Design review of the part built by this model. Coordinates are the model's own, in mm. A direction names the side the tool comes from. Give positions to 0.01 mm unless a question says otherwise; leave off trailing zeros. Write each loop counter-clockwise with the first axis right and the second up, starting at its lowest first coordinate (ties: lowest second). Pieces come first, ordered by that corner, then holes. Notation, with made-up numbers: (60, 77) -> (65, 77) arc R19 ccw to (65, 92) -> close; hole circle Ø6 at (-29.75, 11). An arc over 180 degrees is marked (long way). Return JSON: item names as keys, results as strings. Group by question number.
from build123d import *

# Parameters (mm, degrees)
F0_R     = 1.5
F0_R_2   = 13.666943
F1_DEPTH = 3
F0_W     = 3.25
F0_H     = 5.5
F0_W_2   = 17.75
F2_DEPTH = 45


with BuildPart() as f1:
    # F0 (on Top) → F1 (new body)
    with BuildSketch(Plane.XY):
        Polygon((21, 21), (-21, 21), (-21, -21), (-3.25, -21), (0, -21), (3.25, -21), (21, -21), align=None)
        with Locations((-15.5, -15.5)):
            Circle(F0_R, mode=Mode.SUBTRACT)
        with Locations((15.5, -15.5)):
            Circle(F0_R, mode=Mode.SUBTRACT)
        with Locations((-15.5, 15.5)):
            Circle(F0_R, mode=Mode.SUBTRACT)
        Circle(F0_R_2, mode=Mode.SUBTRACT)
        with Locations((15.5, 15.5)):
            Circle(F0_R, mode=Mode.SUBTRACT)
    extrude(amount=F1_DEPTH)

    # F0 (on Top) → F2 (join)
    with BuildSketch(Plane.XY):
        Polygon((0, -26.5), (-3.25, -26.5), (-3.25, -29.5), (-8.25, -29.5), (-5.5, -34), (0, -34), align=None)
        Polygon((3.25, -29.5), (3.25, -26.5), (0, -26.5), (0, -34), (5.5, -34), (8.25, -29.5), align=None)
        with Locations((1.625, -23.75)):
            Rectangle(F0_W, F0_H)
        with Locations((12.125, -23.75)):
            Rectangle(F0_W_2, F0_H)
        with Locations((-1.625, -23.75)):
            Rectangle(F0_W, F0_H)
        with Locations((-12.125, -23.75)):
            Rectangle(F0_W_2, F0_H)
    extrude(amount=F2_DEPTH)


solid = f1.part
Q1. Tool access review of faces 1 (the face through (-17, -15.43, 1.48)), 2 (the face through (12, -26.5, 22)), 3 (the face through (-12, -26.5, 22)), 4 (the face through (0, 14, 3)): name each direction out of +Z, -Z, +X, -X, +Y, -Y from which nothing blocks a thin tool from reaching the whole face with its end or side.
Q2. Take a section at C-C, the plane x = 0. Give the boundary of the cut face in (y, z), plus the area to 3 significant figures.
Q3. Mouldability with a two-part tool opening along Y and no side actions: class faces 5 (the face through (6.856, -31.782, 22.185)), 6 (the face through (0, -21, 24)), 7 (the face through (-10, -12, 0)), 8 (the face through (3.25, -28, 22)) as +Y half, -Y half, draft (parallel to the pull), parting line (faces both ways), or undercut.
Q4. Take a section at A-A, the plane x = -15.5. Give the boundary of the cut face in (y, z), plus the area to 4 significant figures.
Q5. For L1, parallel to Y at x = -15.5, z = 1.55; L2, parallel to Y at x = -15, z = 1; L3, parallel to X at y = -15, z = 1, list the stretches that pass through material, from the lowest coordinate up. Write a range as from..to.
Q6. Insertion check: pin 1 (2.5 mm diameter, centred on x = 5.5, z = 31.5, fed in from +Y); pin 2 (1.8 mm diameter, centred on x = -15.5, y = -15.5, fed in from -Z); pin 3 (12 mm diameter, centred on x = 9.5, y = 15, fed in from +Z); pin 4 (3.5 mm diameter, centred on x = -15.5, y = 15.5, fed in from -Z). Each pin has a flat end and moves straight along its axis. Give the tip position at first contact, or say it passes through.
Q7. Take a section at B-B, the plane y = -15.5. Give the boundary of the cut face in (x, z).
Q8. Take a section at D-D, the plane z = 14.5. Give the boundary of the cut face in (x, y).
Final values:
{
 "1": {"face 1": "+Z, -Z", "face 2": "+Z, -Z, +X", "face 3": "+Z, -Z, -X", "face 4": "+Z, +X, -X, +Y"},
 "2": {"outline": "(-34, 0) -> (-13.67, 0) -> (-13.67, 3) -> (-21, 3) -> (-21, 45) -> (-34, 45) -> close; (13.67, 0) -> (21, 0) -> (21, 3) -> (13.67, 3) -> close", "area": "629 mm²"},
 "3": {"face 5": "-Y half", "face 6": "+Y half", "face 7": "draft", "face 8": "undercut"},
 "4": {"outline": "(-26.5, 0) -> (-17, 0) -> (-17, 3) -> (-21, 3) -> (-21, 45) -> (-26.5, 45) -> close; (-14, 0) -> (14, 0) -> (14, 3) -> (-14, 3) -> close; (17, 0) -> (21, 0) -> (21, 3) -> (17, 3) -> close", "area": "355.5 mm²"},
 "5": {"L1": "y = -26.5..-17, -14..14, 17..21", "L2": "y = -26.5..-16.91, -14.09..14.09, 16.91..21", "L3": "x = -21..-16.91, -14.09..14.09, 16.91..21"},
 "6": {"pin 1": "stops at y = -21", "pin 2": "passes through", "pin 3": "stops at z = 3", "pin 4": "stops at z = 0"},
 "7": {"outline": "(-21, 0) -> (-17, 0) -> (-17, 3) -> (-21, 3) -> close; (-14, 0) -> (14, 0) -> (14, 3) -> (-14, 3) -> close; (17, 0) -> (21, 0) -> (21, 3) -> (17, 3) -> close"},
 "8": {"outline": "(-21, -26.5) -> (-3.25, -26.5) -> (-3.25, -29.5) -> (-8.25, -29.5) -> (-5.5, -34) -> (5.5, -34) -> (8.25, -29.5) -> (3.25, -29.5) -> (3.25, -26.5) -> (21, -26.5) -> (21, -21) -> (-21, -21) -> close"}
}
